```python
from build123d import *

# Parameters (mm, degrees)
SKETCH1_W           = 40
SKETCH1_H           = 80
BOSS_EXTRUDE1_DEPTH = 100
SKETCH3_R           = 10
SKETCH3_R_2         = 5
CUT_EXTRUDE2_DEPTH  = 20


with BuildPart() as part:
    # Sketch1 → Boss-Extrude1 (new body)
    with BuildSketch(Plane(origin=(0, 0, 0), x_dir=(1, 0, 0), z_dir=(0, 1, 0))):
        Rectangle(SKETCH1_W, SKETCH1_H)
    extrude(amount=BOSS_EXTRUDE1_DEPTH)

    # Sketch3 → Cut-Extrude2 (cut)
    with BuildSketch(Plane.XZ):
        with Locations(Location((0, 0, 0), (0, 0, 270))):
            Circle(SKETCH3_R)
        with Locations(Location((0, 22, 0), (0, 0, 270))):
            Circle(SKETCH3_R_2)
        with Locations(Location((0, -22, 0), (0, 0, 270))):
            Circle(SKETCH3_R_2)
    extrude(amount=-CUT_EXTRUDE2_DEPTH, mode=Mode.SUBTRACT)


solid = part.part
```
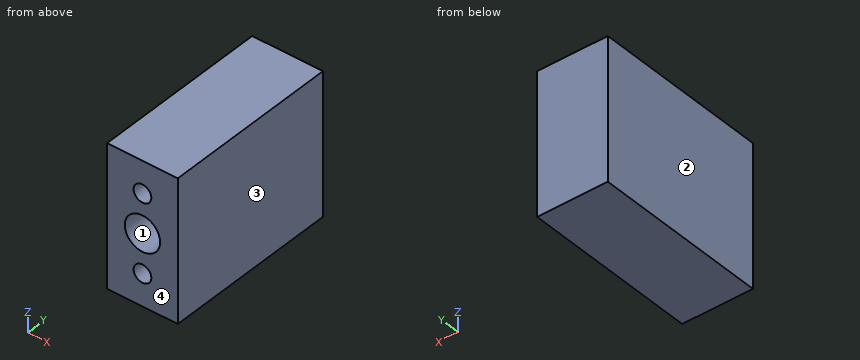
For this review, take the finished solid that the model builds, in its own axes (mm). Face numbers are marked on the shaded views. Give positions to 0.01 mm unless a question says otherwise; leave off trailing zeros. Order: outer loops, then holes, each group sorted by start corner. A loop starts at its lowest first (then second) coordinate and runs counter-clockwise, first axis right, second up.
1) Take a section at A-A (z = 8). Give the boundary of the cut face in (x, y).
2) Insertion check: pin 1 (6 mm diameter, centred on x = -4, z = 2, fed in from -Y); pin 2 (5 mm diameter, centred on x = 2.5, z = 21, fed in from -Y). Each pin has a flat end and moves straight along its axis. Give the tip position at first contact, or say it passes through.
3) Take a section at B-B (x = 0). Give the boundary of the cut face in (y, z).
4) The part is to be moulded in two halves that separate along X. For the marked faces 1, 2, 3 and 4, say which applies: released by +X, released by -X, zero draft, split by the parting line, or undercut.
5) Wall thickness on line 1 (X direction, y = 10.75, z = 0); line 2 (X direction, y = 6, z = -22); line 3 (Z direction, x = -9, y = 13): over which ranges is each line inside the solid? List them lowest first.
6) Take a section at C-C (z = 0). Give the boundary of the cut face in (x, y).
Derived:
1. outline: (-20, 0) - (-6, 0) - (-6, 20) - (6, 20) - (6, 0) - (20, 0) - (20, 100) - (-20, 100) - close
2. pin 1: stops at y = 20
2. pin 2: stops at y = 0
3. outline: (0, -40) - (100, -40) - (100, 40) - (0, 40) - (0, 27) - (20, 27) - (20, 17) - (0, 17) - (0, 10) - (20, 10) - (20, -10) - (0, -10) - (0, -17) - (20, -17) - (20, -27) - (0, -27) - close
4. face 1: undercut
4. face 2: released by -X
4. face 3: released by +X
4. face 4: zero draft
5. line 1: x = -20 to -10, 10 to 20
5. line 2: x = -20 to -5, 5 to 20
5. line 3: z = -40 to -4.36, 4.36 to 40
6. outline: (-20, 0) - (-10, 0) - (-10, 20) - (10, 20) - (10, 0) - (20, 0) - (20, 100) - (-20, 100) - close
